Design review of the part built by this model. Coordinates are the model's own, in mm. A direction names the side the tool comes from. Coordinates: 2 decimals unless noted, no trailing zeros. Loops run counter-clockwise (first coordinate to the right, second up) from the corner with the lowest first, then second, coordinate; pieces in that order, holes last. Notation, with made-up numbers: M 56.5,13 L 109.5,13 A30 cw 109.5,51 Z; hole C 24.5,-17 d10. An arc over 180 degrees is marked long. Put each result on its own line as item: value. Start each with the question number.
(1) Take a section at B-B, the plane x = 156.5. Give the boundary of the cut face in (y, z), then the cut area to 3 significant figures.
(2) Take a section at A-A, the plane y = 16. Give the boundary of the cut face in (x, z), then the cut area to 3 significant figures.
(3) For probe 1 along Z at (x, y) = (690, 20.5); probe 2 along Z at (x, y) = (670, 25); probe 3 along Z at (x, y) = (-632, 21.5), list the stretches that pass through material, from the lowest coordinate up. Write a range as [from, to].
(4) For faces 1 (the flat face through (11, 20, 15)), 2 (the flat face through (-684, 35, -19)), 3 (the flat face through (11, -15, 75)), 4 (the flat face through (685, 35, -29)), 5 (the flat face through (-700, 17, -55)), list the 3-axis set-ups (+Z, -Z, +X, -X, +Y, -Y) from which the entire face can be reached by the end or side of a thin tool; tool diameter is ignored.
(5) Clearance check with flat-ended pins moving along their axes: pin 1 (4 mm diameter, centred on y = 36.5, z = -35, fed in from +X); pin 2 (6 mm diameter, centred on x = 689.5, z = -47.5, fed in from +Y); pin 3 (6 mm diameter, centred on x = 672.5, z = -7.5, fed in from +Y). State where each tip first meets the part, or that it passes through.
```python
from build123d import *

# Parameters (mm, degrees)
F3_DEPTH  = 800
F4_SIZE   = 79.99999
F5_R      = 6
F6_DEPTH  = 50
F7_W      = 116
F7_H      = 90
F8_DEPTH  = 5
F9_R      = 10
F10_W     = 100
F10_H     = 100
F11_DEPTH = 20


# Not quite as in the source:
# - a fillet or chamfer is up to 0.001 mm smaller than in the source, because OpenCascade refuses the exact size


with BuildPart() as f3:
    # F2 (on Right) → F3 (new body, symmetric)
    with BuildSketch(Plane.YZ):
        Polygon((-40, 75), (-40, -75), (40, -75), (40, 15), (0, 15), (0, 75), align=None)
    extrude(amount=F3_DEPTH, both=True)

    # F4 (size 80 in the source; OpenCascade refuses exactly that, so slightly less here)
    f4_edges = [f3.edges().sort_by_distance(p)[0] for p in [
        (800, 40, -30),
        (-800, 40, -30),
    ]]
    chamfer(f4_edges, length=F4_SIZE)

    # F5 (on face) → F6 (cut)
    with BuildSketch(Plane(origin=(0, 40, 0), x_dir=(-1, 0, 0), z_dir=(0, 1, 0))):
        with Locations((-690, -45)):
            Circle(F5_R)
        with Locations((-670, -5)):
            Circle(F5_R)
        with Locations((670, -5)):
            Circle(F5_R)
        with Locations((690, -45)):
            Circle(F5_R)
    extrude(amount=-F6_DEPTH, mode=Mode.SUBTRACT)

    # F7 (on face) → F8 (cut)
    with BuildSketch(Plane(origin=(0, 40, 0), x_dir=(-1, 0, 0), z_dir=(0, 1, 0))):
        with Locations((-702, -30)):
            Rectangle(F7_W, F7_H)
        with Locations((702, -30)):
            Rectangle(F7_W, F7_H)
    extrude(amount=-F8_DEPTH, mode=Mode.SUBTRACT)

    # F9
    f9_edges = [f3.edges().sort_by_distance(p)[0] for p in [
        (0, -40, 75),
    ]]
    fillet(f9_edges, radius=F9_R)

    # F10 (on face) → F11 (cut)
    with BuildSketch(Plane(origin=(0, 0, -75), x_dir=(1, 0, 0), z_dir=(0, 0, -1))):
        with Locations((-710, -50)):
            Rectangle(F10_W, F10_H)
    extrude(amount=-F11_DEPTH, mode=Mode.SUBTRACT)


solid = f3.part
```
Computed values:
1. outline: M -40,-75 L 40,-75 L 40,15 L 0,15 L 0,75 L -30,75 A10 ccw -40,65 Z
1. area: 9,580 mm^2
2. outline: M -744,-55 L -660,-55 L -660,-75 L 744,-75 L 744,15 L -744,15 Z; hole C -690,-45 d12; hole C -670,-5 d12; hole C 670,-5 d12; hole C 690,-45 d12
2. area: 132,000 mm^2
3. probe 1: z = [-75, -51], [-39, 15]
3. probe 2: z = [-75, -11], [1, 15]
3. probe 3: z = [-75, 15]
4. face 1: +Z, +X, -X, +Y
4. face 2: +Z, -Z, -X, +Y
4. face 3: +Z, +X, -X, +Y, -Y
4. face 4: +Z, -Z, +X, +Y
4. face 5: -Z, -X, +Y
5. pin 1: stops at x = 725.5
5. pin 2: stops at y = -10
5. pin 3: stops at y = 35
